Verification items for the finished model (mm, model axes). Face numbers are marked on the shaded views. A direction names the side the tool comes from. Give positions to 0.01 mm unless a question says otherwise; leave off trailing zeros. Loops run counter-clockwise (first coordinate to the right, second up) from the corner with the lowest first, then second, coordinate; pieces in that order, holes last. Notation, with made-up numbers: (-14, -0.5) - (0, -0.5) arc R27 ccw to (0, 37.5) - close; hole circle Ø1 at (83.5, -30). An arc over 180 degrees is marked (long way). Answer in a Markdown table with one row per item.
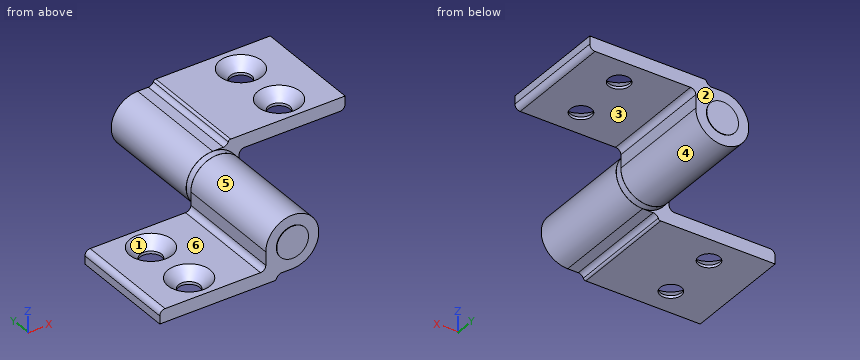
Autodesk Inventor part; units mm, degrees
ref_plane "side_2a_XY" through (-32, -21.925, -19) normal (0, 0, 1) x (1, 0, 0)
ref_plane "side_2a_YZ" through (-32, -21.925, -19) normal (1, 0, 0) x (0, 1, 0)
ref_plane "side_2a_ZX" through (-32, -21.925, -19) normal (0, 1, 0) x (0, 0, 1)
sketch "Skizze_34" plane through (0, 0, 0) normal (0, 1, 0) x (1, 0, 0)
  circle A0 centre (0, 12) radius 10
extrude "Extrusion1" add sketch "Skizze_34" along normal mid plane 2.5
sketch "Skizze_35" plane through (0, 0, 0) normal (0, 1, 0) x (1, 0, 0)
  circle A0 centre (0, 12) radius 6
extrude "Extrusion2" add sketch "Skizze_35" along normal mid plane 85.5
sketch "Skizze_36" plane through (0, -1.3, 0) normal (0, 1, 0) x (1, 0, 0)
  line L0 (-50, 24) -> (-50, 21)
  arc A0 (-50, 21) -> (-48, 19) centre (-48, 21) ccw
  line L1 (-48, 19) -> (-12, 19)
  arc A1 (-10, 17) -> (-12, 19) centre (-12, 17) ccw
  line L2 (-10, 17) -> (-10, 12)
  arc A2 (-10, 12) -> (0, 22) centre (0, 12) ccw
  line L3 (0, 22) -> (-4, 22)
  arc A3 (-5.8856, 23.3333) -> (-4, 22) centre (-4, 24) ccw
  arc A4 (-5.8856, 23.3333) -> (-6.8284, 24) centre (-6.8284, 23) ccw
  line L4 (-6.8284, 24) -> (-50, 24)
  circle A5 centre (0, 12) radius 6
extrude "Extrusion3" add sketch "Skizze_36" against normal blind 41.25
sketch "Skizze_37" plane through (0, 1.3, 0) normal (0, 1, 0) x (1, 0, 0)
  arc A0 (10, 12) -> (0, 2) centre (0, 12) ccw
  line L0 (0, 2) -> (4, 2)
  arc A1 (5.8856, 0.6667) -> (4, 2) centre (4, 0) ccw
  arc A2 (5.8856, 0.6667) -> (6.8284, 0) centre (6.8284, 1) ccw
  line L1 (6.8284, 0) -> (50, 0)
  line L2 (50, 0) -> (50, 3)
  arc A3 (50, 3) -> (48, 5) centre (48, 3) ccw
  line L3 (48, 5) -> (12, 5)
  arc A4 (10, 7) -> (12, 5) centre (12, 7) ccw
  line L4 (10, 7) -> (10, 12)
  circle A5 centre (0, 12) radius 6
extrude "Extrusion4" add sketch "Skizze_37" along normal blind 41.25
sketch "Sketch5" plane through (6.8284, 1.3, 0) normal (0, 0, 1) x (1, 0, 0)
  point P0 (25.1716, 10.13)
hole "Drilling 1" at (32, 11.43, 0) direction (0, 0, -1) diameter 8 depth 5 countersink diameter 16 countersink angle 90
sketch "Sketch6" plane through (6.8284, 1.3, 0) normal (0, 0, 1) x (1, 0, 0)
  point P0 (25.1716, 31.13)
hole "Drilling 2" at (32, 32.43, 0) direction (0, 0, -1) diameter 8 depth 5 countersink diameter 16 countersink angle 90
sketch "Sketch7" plane through (-48, -1.3, -19) normal (0, 0, 1) x (1, 0, 0)
  point P0 (16, -10.13)
hole "Drilling 3" at (-32, -11.43, -19) direction (0, 0, -1) diameter 8 depth 5 countersink diameter 16 countersink angle 90
sketch "Sketch8" plane through (-48, -1.3, -19) normal (0, 0, 1) x (1, 0, 0)
  point P0 (16, -31.13)
hole "Drilling 4" at (-32, -32.43, -19) direction (0, 0, -1) diameter 8 depth 5 countersink diameter 16 countersink angle 90
ref_plane "side_2a_XY" through (-32, -21.925, -19) normal (0, 0, 1) x (1, 0, 0)
ref_plane "side_2a_YZ" through (-32, -21.925, -19) normal (1, 0, 0) x (0, 1, 0)
ref_plane "side_2a_ZX" through (-32, -21.925, -19) normal (0, 1, 0) x (0, 0, 1)
ref_plane "side_2b_XY" through (-32, -21.925, -24) normal (0, 0, -1) x (1, 0, 0)
ref_plane "side_2b_YZ" through (-32, -21.925, -24) normal (1, 0, 0) x (0, -1, 0)
ref_plane "side_2b_ZX" through (-32, -21.925, -24) normal (0, -1, 0) x (0, 0, -1)
ref_plane "side_1b_XY" through (32, 21.925, -5) normal (0, 0, -1) x (-1, 0, 0)
ref_plane "side_1b_YZ" through (32, 21.925, -5) normal (-1, 0, 0) x (0, 1, 0)
ref_plane "side_1b_ZX" through (32, 21.925, -5) normal (0, 1, 0) x (0, 0, -1)
ref_plane "side_3b_XY" through (32, 21.925, -5) normal (0, 0, -1) x (-1, 0, 0)
ref_plane "side_3b_YZ" through (32, 21.925, -5) normal (-1, 0, 0) x (0, 1, 0)
ref_plane "side_3b_ZX" through (32, 21.925, -5) normal (0, 1, 0) x (0, 0, -1)
ref_plane "side_1a_XY" through (32, 21.925, 0) normal (0, 0, 1) x (-1, 0, 0)
ref_plane "side_1a_YZ" through (32, 21.925, 0) normal (-1, 0, 0) x (0, -1, 0)
ref_plane "side_1a_ZX" through (32, 21.925, 0) normal (0, -1, 0) x (0, 0, 1)
ref_plane "side_3a_XY" through (32, 21.925, 0) normal (0, 0, 1) x (-1, 0, 0)
ref_plane "side_3a_YZ" through (32, 21.925, 0) normal (-1, 0, 0) x (0, -1, 0)
ref_plane "side_3a_ZX" through (32, 21.925, 0) normal (0, -1, 0) x (0, 0, 1)
properties part number "MayTec 1.62.842032085_Alu hinges, heavy, type 20 PG 40 (180)"
Q1. Sectioned sample at C-C (y = -21). Record the cut outline in (x, z), and give its area (3 significant figures).
Completed:
| item | result |
|---|---|
| outline | (-50, -24) - (-6.83, -24) arc R1 ccw to (-5.89, -23.33) arc R2 cw to (-4, -22) - (0, -22) arc R10 ccw (long way) to (-10, -12) - (-10, -17) arc R2 cw to (-12, -19) - (-48, -19) arc R2 ccw to (-50, -21) - close |
| area | 544 mm^2 |
Q2. Sectioned sample at B-B (y = -32.43). Record the cut outline in (x, z), and give its area (3 significant figures).
Completed:
| item | result |
|---|---|
| outline | (-50, -24) - (-36, -24) - (-36, -23) - (-40, -19) - (-48, -19) arc R2 ccw to (-50, -21) - close; (-28, -24) - (-6.83, -24) arc R1 ccw to (-5.89, -23.33) arc R2 cw to (-4, -22) - (0, -22) arc R10 ccw (long way) to (-10, -12) - (-10, -17) arc R2 cw to (-12, -19) - (-24, -19) - (-28, -23) - close |
| area | 488 mm^2 |
Q3. Sectioned sample at A-A (x = 32). Record the cut outline in (y, z).
Completed:
| item | result |
|---|---|
| outline | (1.3, -5) - (7.43, -5) - (7.43, -4) - (3.43, 0) - (1.3, 0) - close; (15.43, -5) - (28.43, -5) - (28.43, -4) - (24.43, 0) - (19.43, 0) - (15.43, -4) - close; (36.43, -5) - (42.55, -5) - (42.55, 0) - (40.43, 0) - (36.43, -4) - close |
Q4. Draft check along Y on the marked faces 1, 2 and 3. Enter one of: +Y half, -Y half, draft (parallel to the pull), parting line (faces both ways), or undercut.
Completed:
| item | result |
|---|---|
| face 1 | undercut |
| face 2 | +Y half |
| face 3 | draft |
Q5. Thickness scan on line 1 (Y direction, x = -32, z = -23.55); line 2 (Y direction, x = 32, z = -4.5); line 3 (X direction, y = -11.43, z = -23.4). Record the ranges inside material, lowest first.
Completed:
| item | result |
|---|---|
| line 1 | -42.55 to -36.43, -28.43 to -15.43, -7.43 to -1.3 |
| line 2 | 1.3 to 7.43, 15.43 to 28.43, 36.43 to 42.55 |
| line 3 | -50 to -36, -28 to -5.91 |
Q6. Sectioned sample at D-D (z = -9). Record the cut outline in (x, y).
Completed:
| item | result |
|---|---|
| outline | (-9.54, -42.55) - (-5.2, -42.55) - (-5.2, -42.75) - (5.2, -42.75) - (5.2, -42.55) - (9.54, -42.55) - (9.54, -1.3) - (5.2, -1.3) - (5.2, -1.25) - (9.54, -1.25) - (9.54, 1.25) - (5.2, 1.25) - (5.2, 1.3) - (10, 1.3) - (10, 42.55) - (5.2, 42.55) - (5.2, 42.75) - (-5.2, 42.75) - (-5.2, 42.55) - (-9.54, 42.55) - (-9.54, 1.3) - (-5.2, 1.3) - (-5.2, 1.25) - (-9.54, 1.25) - (-9.54, -1.25) - (-5.2, -1.25) - (-5.2, -1.3) - (-9.54, -1.3) - close |
Q7. Go/stop test with flat-tipped pins: P1, Ø12, axis at y = -18.5, z = -8.5, coming from the +X side; P2, Ø2, axis at y = 14, z = -19, coming from the -X side; P3, Ø2.5, axis at y = -23, z = -14, coming from the -X side; P4, Ø7, axis at x = -32, y = -32.43, coming from the +Z side. Record where each tip stops, or that it passes through.
Completed:
| item | result |
|---|---|
| P1 | x = 10 |
| P2 | x = -8 |
| P3 | x = -10 |
| P4 | through |
Q8. Tool access check on the marked faces 4, 5 and 6. Record the directions out of +Z, -Z, +X, -X, +Y, -Y that give a thin tool (end or side, any length) a straight path to the whole face; none if there is none.
Completed:
| item | result |
|---|---|
| face 4 | +Y |
| face 5 | -Y |
| face 6 | +Z, -X, +Y, -Y |
